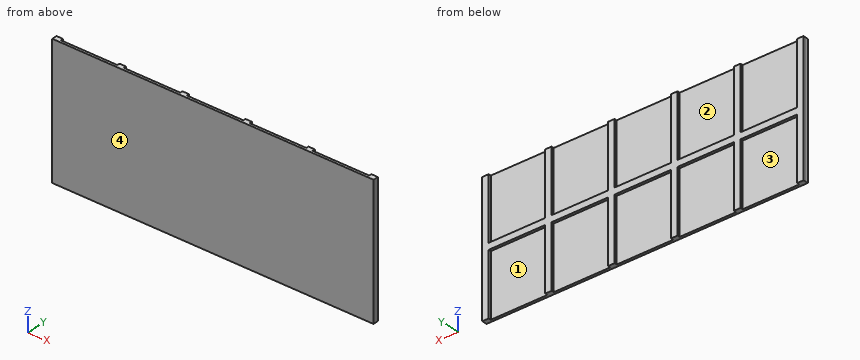
```python
from build123d import *

# Parameters (mm, degrees)
BOSS_EXTRUDE1_DEPTH = 10
SKETCH2_W           = 1250.061929379
SKETCH2_H           = 515
BOSS_EXTRUDE2_DEPTH = 10


with BuildPart() as part:
    # Sketch1 → Boss-Extrude1 (new body)
    with BuildSketch(Plane(origin=(0, 0, 0), x_dir=(1, 0, 0), z_dir=(0, 1, 0))):
        Polygon((-110, 128.75), (-135, 128.75), (-135, -116.25), (-355, -116.25), (-355, 128.75), (-380, 128.75), (-380, -116.25), (-600, -116.25), (-600, 128.75), (-625, 128.75), (-625, -386.25), (-600, -386.25), (-600, -141.25), (-380, -141.25), (-380, -386.25), (-355, -386.25), (-355, -141.25), (-135, -141.25), (-135, -386.25), (-110, -386.25), (-110, -141.25), (110, -141.25), (110, -386.25), (135, -386.25), (135, -141.25), (355, -141.25), (355, -386.25), (380, -386.25), (380, -141.25), (600, -141.25), (600, -386.25), (625, -386.25), (625, 128.75), (600, 128.75), (600, -116.25), (380, -116.25), (380, 128.75), (355, 128.75), (355, -116.25), (135, -116.25), (135, 128.75), (110, 128.75), (110, -116.25), (-110, -116.25), align=None)
    extrude(amount=BOSS_EXTRUDE1_DEPTH)

    # Sketch2 → Boss-Extrude2 (add)
    with BuildSketch(Plane(origin=(0, 0, 0), x_dir=(1, 0, 0), z_dir=(0, 1, 0))):
        with Locations((-0.03096469, -128.75)):
            Rectangle(SKETCH2_W, SKETCH2_H)
    extrude(amount=-BOSS_EXTRUDE2_DEPTH)


solid = part.part
```
Geometry check sheet. Reference: the model listing, model coordinates, mm. Face numbers are marked on the shaded views. A direction names the side the tool comes from. Coordinates: 2 decimals unless noted, no trailing zeros. Loops run counter-clockwise (first coordinate to the right, second up) from the corner with the lowest first, then second, coordinate; pieces in that order, holes last. Notation, with made-up numbers: (-22, 9) -> (4, 9) arc R26 cw to (4, 46) -> close; hole circle Ø1 at (-38, 42). An arc over 180 degrees is marked (long way). Put each result on its own line as item: value.
1) Cross-section at B-B on z = -0.5. Record the boundary of the cut face in (x, y), plus the area to 3 significant figures.
Result set:
outline: (-625.06, -10) -> (625, -10) -> (625, 10) -> (600, 10) -> (600, 0) -> (380, 0) -> (380, 10) -> (355, 10) -> (355, 0) -> (135, 0) -> (135, 10) -> (110, 10) -> (110, 0) -> (-110, 0) -> (-110, 10) -> (-135, 10) -> (-135, 0) -> (-355, 0) -> (-355, 10) -> (-380, 10) -> (-380, 0) -> (-600, 0) -> (-600, 10) -> (-625, 10) -> (-625, 0) -> (-625.06, 0) -> close
area: 14,000 mm^2
2) Cross-section at A-A on x = 293.5. Record the boundary of the cut face in (y, z), plus the area to 3 significant figures.
Result set:
outline: (-10, -128.75) -> (0, -128.75) -> (0, 116.25) -> (10, 116.25) -> (10, 141.25) -> (0, 141.25) -> (0, 386.25) -> (-10, 386.25) -> close
area: 5,400 mm^2
3) Release check for a two-part mould opening along X. For the marked faces 3 and 4 record: released by +X, released by -X, zero draft, split by the parting line, or undercut.
Result set:
face 3: undercut
face 4: zero draft
4) Tool access check on the marked faces 1 and 2. Record the directions out of +Z, -Z, +X, -X, +Y, -Y that give a thin tool (end or side, any length) a straight path to the whole face; none if there is none.
Result set:
face 1: -Z, +Y
face 2: +Z, +Y
5) Thickness scan on line 1 (X direction, y = 8.5, z = -60.5); line 2 (Z direction, x = 151, y = 7.25); line 3 (Y direction, x = -74.5, z = 248). Record the ranges inside material, lowest first.
Result set:
line 1: x = -625 to -600, -380 to -355, -135 to -110, 110 to 135, 355 to 380, 600 to 625
line 2: z = 116.25 to 141.25
line 3: y = -10 to 0
6) Gauge pin test, flat ends, axial feed: pin 1 Ø11 at (x, y) = (-39.5, 6.5) entering from +Z; pin 2 Ø5 at (x, y) = (8.5, 6) entering from -Z; pin 3 Ø1.5 at (x, z) = (237.5, 197.5) entering from +Y. Record the tip position at first contact, or that the pin passes through.
Result set:
pin 1: stops at z = 141.25
pin 2: stops at z = 116.25
pin 3: stops at y = 0
